```python
from build123d import *

# Parameters (mm, degrees)
SKETCH1_W           = 82.9
SKETCH1_H           = 83.7
SKETCH1_R           = 3
SKETCH1_W_2         = 62.9
SKETCH1_H_2         = 63.7
BOSS_EXTRUDE1_DEPTH = 13
SKETCH1_4_W         = 62.9
SKETCH1_4_H         = 63.7
BOSS_EXTRUDE2_DEPTH = 3
SKETCH2_W           = 18.5
SKETCH2_H           = 10
CUT_EXTRUDE1_DEPTH  = 7.5
FILLET1_R           = 5


with BuildPart() as part:
    # Sketch1 → Boss-Extrude1 (new body)
    with BuildSketch(Plane(origin=(0, 0, 0), x_dir=(1, 0, 0), z_dir=(0, 1, 0))):
        with Locations((-33.914696313, -1.170240017)):
            Rectangle(SKETCH1_W, SKETCH1_H)
        with Locations(Location((2.535303687, -38.020240017, 0), (0, 0, 90))):
            Circle(SKETCH1_R, mode=Mode.SUBTRACT)
        with Locations(Location((-70.364696313, -38.020240017, 0), (0, 0, 90))):
            Circle(SKETCH1_R, mode=Mode.SUBTRACT)
        with Locations(Location((-70.364696313, 35.679759983, 0), (0, 0, 90))):
            Circle(SKETCH1_R, mode=Mode.SUBTRACT)
        with Locations(Location((2.535303687, 35.679759983, 0), (0, 0, 90))):
            Circle(SKETCH1_R, mode=Mode.SUBTRACT)
        with Locations((-33.914696313, -1.170240017)):
            Rectangle(SKETCH1_W_2, SKETCH1_H_2, mode=Mode.SUBTRACT)
    extrude(amount=BOSS_EXTRUDE1_DEPTH)

    # Sketch1_4 → Boss-Extrude2 (add)
    with BuildSketch(Plane(origin=(0, 0, 0), x_dir=(1, 0, 0), z_dir=(0, 1, 0))):
        with Locations((-33.914696313, -1.170240017)):
            Rectangle(SKETCH1_4_W, SKETCH1_4_H)
    extrude(amount=BOSS_EXTRUDE2_DEPTH)

    # Sketch2 → Cut-Extrude1 (cut)
    with BuildSketch(Plane(origin=(0, 13, 0), x_dir=(1, 0, 0), z_dir=(0, 1, 0))):
        with Locations((-33.914696313, 35.679759983)):
            Rectangle(SKETCH2_W, SKETCH2_H)
    extrude(amount=-CUT_EXTRUDE1_DEPTH, mode=Mode.SUBTRACT)

    # Fillet1
    fillet1_edges = [part.edges().sort_by_distance(p)[0] for p in [
        (7.535303687, 6.5, 43.020240017),
        (-75.364696313, 6.5, 43.020240017),
        (-75.364696313, 6.5, -40.679759983),
        (7.535303687, 6.5, -40.679759983),
    ]]
    fillet(fillet1_edges, radius=FILLET1_R)


solid = part.part
```
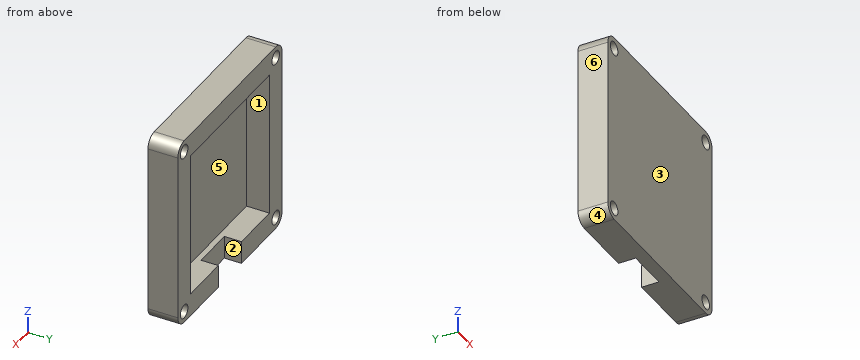
Geometry check sheet. Reference: the model listing, model coordinates, mm. Face numbers are marked on the shaded views. A direction names the side the tool comes from. Coordinates: 2 decimals unless noted, no trailing zeros. Write each loop counter-clockwise with the first axis right and the second up, starting at its lowest first coordinate (ties: lowest second). Pieces come first, ordered by that corner, then holes. Notation, with made-up numbers: M 50.25,16 L 59.25,16 A25 ccw 59.25,42 Z; hole C 88,-30 d4. An arc over 180 degrees is marked long. One line per item, written item: value. Start each with the question number.
(1) Release check for a two-part mould opening along X. For the marked faces 1, 2, 3 and 4 record: released by +X, released by -X, zero draft, split by the parting line, or undercut.
(2) Tool access check on the marked faces 5 and 6. Record the directions out of +Z, -Z, +X, -X, +Y, -Y that give a thin tool (end or side, any length) a straight path to the whole face; none if there is none.
(3) Sectioned sample at B-B, the plane y = 4. Enter the section's corners in (x, z).
(4) Scan lines: line 1 along X through (y, z) = (6.5, 38); line 2 along X through (y, z) = (10.25, 24); line 3 along Z through (x, y) = (-61.5, 5.5). Record each from-to range of solid material in increasing order. Write a range as [from, to].
(5) Sectioned sample at C-C, the plane z = -0.5. Enter the section's corners in (x, y).
(6) Depth check by flat-ended pin: pin 1 (5 mm diameter, centred on x = -33, z = -37.5, fed in from +Y); pin 2 (2 mm diameter, centred on x = -39, z = 6.5, fed in from +Y). Enter the tip coordinate at first touch or a pass-through.
(7) Sectioned sample at A-A, the plane x = -61.5. Enter the section's corners in (y, z), and give its area (3 significant figures).
(8) Sectioned sample at D-D, the plane y = 11.25. Enter the section's corners in (x, z).
Filled sheet:
1. face 1: undercut
1. face 2: undercut
1. face 3: zero draft
1. face 4: released by -X
2. face 5: +Y
2. face 6: +Z, -Z, -X, +Y, -Y
3. outline: M -75.36,-35.68 A5 ccw -70.36,-40.68 L 2.54,-40.68 A5 ccw 7.54,-35.68 L 7.54,38.02 A5 ccw 2.54,43.02 L -70.36,43.02 A5 ccw -75.36,38.02 Z; hole C -70.36,-35.68 d6; hole C -70.36,38.02 d6; hole M -65.36,-30.68 L -2.46,-30.68 L -2.46,33.02 L -65.36,33.02 Z; hole C 2.54,-35.68 d6; hole C 2.54,38.02 d6
4. line 1: [-75.36, -73.36], [-67.36, -0.46], [5.54, 7.54]
4. line 2: [-75.36, -65.36], [-2.46, 7.54]
4. line 3: [-40.68, -30.68], [33.02, 43.02]
5. outline: M -75.36,0 L 7.54,0 L 7.54,13 L -2.46,13 L -2.46,3 L -65.36,3 L -65.36,13 L -75.36,13 Z
6. pin 1: y = 5.5
6. pin 2: y = 3
7. outline: M 0,-40.68 L 13,-40.68 L 13,-30.68 L 3,-30.68 L 3,33.02 L 13,33.02 L 13,43.02 L 0,43.02 Z
7. area: 451 mm²
8. outline: M -75.36,-35.68 A5 ccw -70.36,-40.68 L -43.16,-40.68 L -43.16,-30.68 L -65.36,-30.68 L -65.36,33.02 L -2.46,33.02 L -2.46,-30.68 L -24.66,-30.68 L -24.66,-40.68 L 2.54,-40.68 A5 ccw 7.54,-35.68 L 7.54,38.02 A5 ccw 2.54,43.02 L -70.36,43.02 A5 ccw -75.36,38.02 Z; hole C -70.36,-35.68 d6; hole C -70.36,38.02 d6; hole C 2.54,-35.68 d6; hole C 2.54,38.02 d6
